Input: part model. Units: mm. Frame: model coordinates. A direction names the side the tool comes from. Coordinates: 2 decimals unless noted, no trailing zeros. Order: outer loops, then holes, each group sorted by start corner. A loop starts at its lowest first (then second) coordinate and runs counter-clockwise, first axis right, second up. Notation, with made-up numbers: (-9.75, 54) -> (27.25, 54) arc R22 cw to (27.25, 92) -> close; hole circle Ø1 at (0, -22.5). An arc over 180 degrees is marked (long way). Write each question's results on one line, items separated by ' | '.
```python
from build123d import *

# Parameters (mm, degrees)
F0_W     = 609.6
F0_H     = 914.4
F1_DEPTH = 914.4
F3_DEPTH = 889
F4_R     = 25.4
F5_DEPTH = 914.401


with BuildPart() as f1:
    # F0 (on Top) → F1 (new body)
    with BuildSketch(Plane.XY):
        with Locations((304.8, -457.2)):
            Rectangle(F0_W, F0_H)
    extrude(amount=-F1_DEPTH)

    # F2 (on face) → F3 (cut)
    with BuildSketch(Plane(origin=(0, 0, -914.4), x_dir=(1, 0, 0), z_dir=(0, 0, -1))):
        Polygon((50.8, 50.8), (50.8, 0), (558.8, 0), (558.8, 50.8), (609.6, 50.8), (609.6, 863.6), (558.8, 863.6), (558.8, 914.4), (50.8, 914.4), (50.8, 863.6), (0, 863.6), (0, 50.8), align=None)
    extrude(amount=-F3_DEPTH, mode=Mode.SUBTRACT)

    # F4 (on face) → F5 (cut, through all)
    with BuildSketch(Plane.XY):
        with Locations((101.6, -101.6)):
            Circle(F4_R)
        with Locations((203.2, -101.6)):
            Circle(F4_R)
        with Locations((304.8, -101.6)):
            Circle(F4_R)
        with Locations((406.4, -101.6)):
            Circle(F4_R)
        with Locations((508, -101.6)):
            Circle(F4_R)
        with Locations((508, -203.2)):
            Circle(F4_R)
        with Locations((406.4, -203.2)):
            Circle(F4_R)
        with Locations((304.8, -203.2)):
            Circle(F4_R)
        with Locations((203.2, -203.2)):
            Circle(F4_R)
        with Locations((101.6, -203.2)):
            Circle(F4_R)
        with Locations((101.6, -304.8)):
            Circle(F4_R)
        with Locations((203.2, -304.8)):
            Circle(F4_R)
        with Locations((304.8, -304.8)):
            Circle(F4_R)
        with Locations((406.4, -304.8)):
            Circle(F4_R)
        with Locations((508, -304.8)):
            Circle(F4_R)
        with Locations((508, -406.4)):
            Circle(F4_R)
        with Locations((406.4, -406.4)):
            Circle(F4_R)
        with Locations((304.8, -406.4)):
            Circle(F4_R)
        with Locations((203.2, -406.4)):
            Circle(F4_R)
        with Locations((101.6, -406.4)):
            Circle(F4_R)
        with Locations((101.6, -508)):
            Circle(F4_R)
        with Locations((203.2, -508)):
            Circle(F4_R)
        with Locations((304.8, -508)):
            Circle(F4_R)
        with Locations((406.4, -508)):
            Circle(F4_R)
        with Locations((508, -508)):
            Circle(F4_R)
        with Locations((508, -609.6)):
            Circle(F4_R)
        with Locations((406.4, -609.6)):
            Circle(F4_R)
        with Locations((304.8, -609.6)):
            Circle(F4_R)
        with Locations((203.2, -609.6)):
            Circle(F4_R)
        with Locations((101.6, -609.6)):
            Circle(F4_R)
        with Locations((101.6, -711.2)):
            Circle(F4_R)
        with Locations((203.2, -711.2)):
            Circle(F4_R)
        with Locations((304.8, -711.2)):
            Circle(F4_R)
        with Locations((406.4, -711.2)):
            Circle(F4_R)
        with Locations((508, -711.2)):
            Circle(F4_R)
        with Locations((508, -812.8)):
            Circle(F4_R)
        with Locations((406.4, -812.8)):
            Circle(F4_R)
        with Locations((304.8, -812.8)):
            Circle(F4_R)
        with Locations((203.2, -812.8)):
            Circle(F4_R)
        with Locations((101.6, -812.8)):
            Circle(F4_R)
    extrude(amount=-F5_DEPTH, mode=Mode.SUBTRACT)


solid = f1.part
```
(1) Reachability of faces 1 (the face through (532.227, -195.571, -12.522)), 2 (the face through (50.8, -889, -476)) from +Z, -Z, +X, -X, +Y, -Y: full face, straight path, thin tool, end or side. Return the list, or none.
Return value:
face 1: +Z, -Z | face 2: -Z, +Y, -Y
(2) Cut plane A-A, the plane y = -609.6. Return loops of the section in (x, z), plus the area to 3 significant figures.
Return value:
outline: (0, -25.4) -> (76.2, -25.4) -> (76.2, 0) -> (0, 0) -> close; (127, -25.4) -> (177.8, -25.4) -> (177.8, 0) -> (127, 0) -> close; (228.6, -25.4) -> (279.4, -25.4) -> (279.4, 0) -> (228.6, 0) -> close; (330.2, -25.4) -> (381, -25.4) -> (381, 0) -> (330.2, 0) -> close; (431.8, -25.4) -> (482.6, -25.4) -> (482.6, 0) -> (431.8, 0) -> close; (533.4, -25.4) -> (609.6, -25.4) -> (609.6, 0) -> (533.4, 0) -> close | area: 9,030 mm2
(3) Mould query, pull axis X, two halves, no side actions, for faces 3 (the face through (584, -50.8, -476)), 4 (the face through (418.121, -835.334, -12.522)). Classes: +X half, -X half, draft (parallel to the pull), parting line (faces both ways), or undercut.
Return value:
face 3: draft | face 4: undercut
(4) Line query: line 1 along X through (y, z) = (-872.5, -381); line 2 along Y through (x, z) = (47, -594); line 3 along Z through (x, y) = (556.5, -506). Output: solid intervals per line, ascending. Write a range as from..to.
Return value:
line 1: 0..50.8, 558.8..609.6 | line 2: -914.4..-863.6, -50.8..0 | line 3: -25.4..0
(5) Pin query (flat end, axial travel): P1, Ø8, axis at x = 418.5, y = -452, coming from the +Z side; P2, Ø8, axis at x = 169.5, y = -804, coming from the -Z side. Return the tip coordinate at first contact, or that it passes through.
Return value:
P1: z = 0 | P2: z = -25.4
(6) Cut plane C-C, the plane x = 508. Count the separate pieces of the cut face and the enclosed holes in it, plus the area to 3 significant figures.
Return value:
separate pieces: 9 | enclosed holes: 0 | area: 12,900 mm2
(7) Cut plane B-B, the plane z = -320. Return loops of the section in (x, y).
Return value:
outline: (0, -914.4) -> (50.8, -914.4) -> (50.8, -863.6) -> (0, -863.6) -> close; (0, -50.8) -> (50.8, -50.8) -> (50.8, 0) -> (0, 0) -> close; (558.8, -914.4) -> (609.6, -914.4) -> (609.6, -863.6) -> (558.8, -863.6) -> close; (558.8, -50.8) -> (609.6, -50.8) -> (609.6, 0) -> (558.8, 0) -> close
